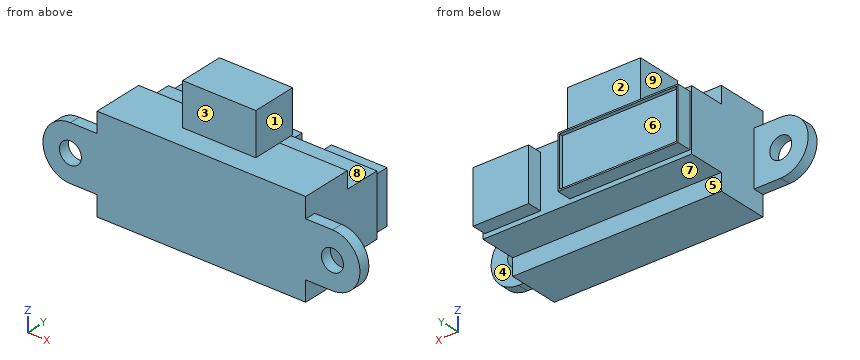
```python
from build123d import *

# Parameters (mm, degrees)
SKETCH1_W           = 28.5
SKETCH1_H           = 13
BOSS_EXTRUDE1_DEPTH = 7
SKETCH2_W           = 28.5
SKETCH2_H           = 8.4
BOSS_EXTRUDE2_DEPTH = 5
SKETCH4_W           = 16.4
SKETCH4_H           = 7.2
SKETCH4_W_2         = 7.6
BOSS_EXTRUDE3_DEPTH = 2
SKETCH5_W           = 16
SKETCH5_H           = 6.8
CUT_EXTRUDE1_DEPTH  = 0.5
SKETCH6_R           = 1.5
BOSS_EXTRUDE4_DEPTH = 1.5
SKETCH7_W           = 10
SKETCH7_H           = 5.8
BOSS_EXTRUDE5_DEPTH = 6.2


with BuildPart() as part:
    # Sketch1 → Boss-Extrude1 (new body)
    with BuildSketch(Plane(origin=(0, 0, 0), x_dir=(1, 0, 0), z_dir=(0, 1, 0))):
        Rectangle(SKETCH1_W, SKETCH1_H)
    extrude(amount=BOSS_EXTRUDE1_DEPTH)

    # Sketch2 → Boss-Extrude2 (add)
    with BuildSketch(Plane(origin=(0, 7, 0), x_dir=(1, 0, 0), z_dir=(0, 1, 0))):
        Rectangle(SKETCH2_W, SKETCH2_H)
    extrude(amount=BOSS_EXTRUDE2_DEPTH)

    # Sketch4 → Boss-Extrude3 (add)
    with BuildSketch(Plane(origin=(0, 12, 0), x_dir=(1, 0, 0), z_dir=(0, 1, 0))):
        with Locations((-5.8, 0)):
            Rectangle(SKETCH4_W, SKETCH4_H)
        with Locations((10.2, 0)):
            Rectangle(SKETCH4_W_2, SKETCH4_H)
    extrude(amount=BOSS_EXTRUDE3_DEPTH)

    # Sketch5 → Cut-Extrude1 (cut)
    with BuildSketch(Plane(origin=(0, 14, 0), x_dir=(1, 0, 0), z_dir=(0, 1, 0))):
        with Locations((-5.8, 0)):
            Rectangle(SKETCH5_W, SKETCH5_H)
    extrude(amount=-CUT_EXTRUDE1_DEPTH, mode=Mode.SUBTRACT)

    # Sketch6 → Boss-Extrude4 (add)
    with BuildSketch(Plane(origin=(0, 0, 0), x_dir=(1, 0, 0), z_dir=(0, 1, 0))):
        with BuildLine():
            Line((-14.25, 3.75), (-14.25, -3.75))
            Line((-14.25, -3.75), (-17.9, -3.75))
            ThreePointArc((-17.9, -3.75), (-21.65, 0), (-17.9, 3.75))
            Line((-17.9, 3.75), (-14.25, 3.75))
        make_face()
        with Locations((-17.9, 0)):
            Circle(SKETCH6_R, mode=Mode.SUBTRACT)
    boss_extrude4 = extrude(amount=BOSS_EXTRUDE4_DEPTH)

    # Mirror1: Boss-Extrude4 across plane
    add(boss_extrude4.mirror(Plane(origin=(0, 0, 0), x_dir=(0, 0, 1), z_dir=(1, 0, 0))))

    # Sketch7 → Boss-Extrude5 (add)
    with BuildSketch(Plane(origin=(0, 3, 0), x_dir=(1, 0, 0), z_dir=(0, 1, 0))):
        with Locations((0, -9.4)):
            Rectangle(SKETCH7_W, SKETCH7_H)
    extrude(amount=BOSS_EXTRUDE5_DEPTH)


solid = part.part
```
Work out the finished part from the listing and answer in its coordinate system (mm). Face numbers are marked on the shaded views. A direction names the side the tool comes from. Coordinates: 2 decimals unless noted, no trailing zeros. Write each loop counter-clockwise with the first axis right and the second up, starting at its lowest first coordinate (ties: lowest second). Pieces come first, ordered by that corner, then holes.
Q1. A cutting plane is placed at D-D, the plane y = 4. Give the vertices of the cut face in (x, z).
Q2. A cutting plane is placed at B-B, the plane z = 0. Give the vertices of the cut face in (x, y).
Q3. Find the intervals of material crossed by line 1 (X direction, y = 0.85, z = 0); line 2 (Z direction, x = 17.9, y = 0.8), in increasing order.
Q4. A cutting plane is placed at C-C, the plane x = -6.5. Give the vertices of the cut face in (y, z), then the cut area to 3 significant figures.
Q5. Determine the mould class of the marked faces 6, 7, 8 and 9 for opening direction Z: released by +Z, released by -Z, zero draft, split by the parting line, or undercut.
Q6. A cutting plane is placed at A-A, the plane y = 12.75. Give the vertices of the cut face in (x, z), then the cut area to 3 significant figures.
Q7. Each of these flat-tipped pins is pushed along its axis until it touches: pin 1 Ø0.6 at (y, z) = (12.5, -1.5) entering from -X; pin 2 Ø2 at (y, z) = (12.5, 1) entering from +X; pin 3 Ø1.5 at (y, z) = (8.5, 4.5) entering from -X. Where does it stop, or does it pass through?
Q8. Which of the six approach directions +Z, -Z, +X, -X, +Y, -Y give full straight-line access (tool end or side, diameter ignored) to the marked faces 1, 2, 3, 4 and 5?
Findings below:
1. outline: (-14.25, -6.5) - (14.25, -6.5) - (14.25, 6.5) - (5, 6.5) - (5, 12.3) - (-5, 12.3) - (-5, 6.5) - (-14.25, 6.5) - close
2. outline: (-21.65, 0) - (-19.4, 0) - (-19.4, 1.5) - (-21.65, 1.5) - close; (-16.4, 0) - (16.4, 0) - (16.4, 1.5) - (14.25, 1.5) - (14.25, 12) - (14, 12) - (14, 14) - (6.4, 14) - (6.4, 12) - (2.4, 12) - (2.4, 14) - (2.2, 14) - (2.2, 13.5) - (-13.8, 13.5) - (-13.8, 14) - (-14, 14) - (-14, 12) - (-14.25, 12) - (-14.25, 1.5) - (-16.4, 1.5) - close; (19.4, 0) - (21.65, 0) - (21.65, 1.5) - (19.4, 1.5) - close
3. line 1: x = -21.65 to -19.4, -16.4 to 16.4, 19.4 to 21.65
3. line 2: z = -3.75 to -1.5, 1.5 to 3.75
4. outline: (0, -6.5) - (7, -6.5) - (7, -4.2) - (12, -4.2) - (12, -3.6) - (14, -3.6) - (14, -3.4) - (13.5, -3.4) - (13.5, 3.4) - (14, 3.4) - (14, 3.6) - (12, 3.6) - (12, 4.2) - (7, 4.2) - (7, 6.5) - (0, 6.5) - close
4. area: 144 mm2
5. face 6: undercut
5. face 7: released by -Z
5. face 8: undercut
5. face 9: zero draft
6. outline: (-14, -3.6) - (2.4, -3.6) - (2.4, 3.6) - (-14, 3.6) - close; (6.4, -3.6) - (14, -3.6) - (14, 3.6) - (6.4, 3.6) - close
6. area: 173 mm2
7. pin 1: stops at x = -14
7. pin 2: stops at x = 14.25
7. pin 3: stops at x = -14.25
8. face 1: +Z, +X, +Y, -Y
8. face 2: +Z, +X, -X, +Y
8. face 3: +Z, +X, -X, -Y
8. face 4: +Z, -Z, +X, +Y
8. face 5: -Z, +X, -X, +Y
